```python
from build123d import *

# Parameters (mm, degrees)
SKETCH1_R           = 5.075
BOSS_EXTRUDE1_DEPTH = 20
CHAMFER1_SIZE       = 1
FILLET1_R           = 5
SKETCH2_R           = 1.5
CUT_EXTRUDE1_DEPTH  = 15
CHAMFER2_SIZE       = 1


with BuildPart() as part:
    # Sketch1 → Boss-Extrude1 (new body)
    with BuildSketch(Plane(origin=(0, 0, 0), x_dir=(0, 0, -1), z_dir=(1, 0, 0))):
        Polygon((0, 0), (60, 0), (60, 15), (45, 15), (45, 196.075), (15, 196.075), (15, 15), (0, 15), align=None)
        with Locations((30, 184.575)):
            Circle(SKETCH1_R, mode=Mode.SUBTRACT)
        with Locations((30, 167.575)):
            Circle(SKETCH1_R, mode=Mode.SUBTRACT)
    extrude(amount=BOSS_EXTRUDE1_DEPTH)

    # Chamfer1
    chamfer1_edges = [part.edges().sort_by_distance(p)[0] for p in [
        (10, 15, 0),
        (10, 196.075, -15),
        (10, 196.075, -45),
        (10, 15, -60),
    ]]
    chamfer(chamfer1_edges, length=CHAMFER1_SIZE)

    # Fillet1
    fillet1_edges = [part.edges().sort_by_distance(p)[0] for p in [
        (10, 15, -15),
        (10, 15, -45),
    ]]
    fillet(fillet1_edges, radius=FILLET1_R)

    # Sketch2 → Cut-Extrude1 (cut)
    with BuildSketch(Plane(origin=(0, 15, 0), x_dir=(1, 0, 0), z_dir=(0, 1, 0))):
        with Locations(Location((5.5, 54.5, 0), (0, 0, 270))):
            Circle(SKETCH2_R)
        with Locations(Location((14.5, 54.5, 0), (0, 0, 270))):
            Circle(SKETCH2_R)
        with Locations(Location((5.5, 5.5, 0), (0, 0, 270))):
            Circle(SKETCH2_R)
        with Locations(Location((14.5, 5.5, 0), (0, 0, 270))):
            Circle(SKETCH2_R)
    extrude(amount=-CUT_EXTRUDE1_DEPTH, mode=Mode.SUBTRACT)

    # Chamfer2
    chamfer2_edges = [part.edges().sort_by_distance(p)[0] for p in [
        (14.5, 15, -56),
        (5.5, 15, -7),
        (14.5, 15, -7),
        (5.5, 15, -56),
    ]]
    chamfer(chamfer2_edges, length=CHAMFER2_SIZE)


solid = part.part
```
Verification items for the finished model (mm, model axes). A direction names the side the tool comes from. Round coordinates to 2 decimals unless told otherwise and drop trailing zeros. Write each loop counter-clockwise with the first axis right and the second up, starting at its lowest first coordinate (ties: lowest second). Pieces come first, ordered by that corner, then holes. Notation, with made-up numbers: (89.5, 27.5) -> (140.5, 27.5) arc R5 cw to (140.5, 31.5) -> close; hole circle Ø2 at (53, 22.5). An arc over 180 degrees is marked (long way). Write each question's results on one line, items separated by ' | '. Start each with the question number.
1. Depth check by flat-ended pin: P1, Ø10, axis at x = 9, y = 142.5, coming from the -Z side; P2, Ø7, axis at x = 14, z = -53, coming from the +Y side; P3, Ø10, axis at x = 15, y = 79.5, coming from the +Z side; P4, Ø2.5, axis at x = 5.5, z = -5.5, coming from the -Y side (1 decimal). Enter the tip coordinate at first touch or a pass-through.
2. Cross-section at C-C (z = -47). Enter the section's corners in (x, y), then the cut area to 3 significant figures.
3. Set-up check for faces 1 (the flat face through (10, 106, -45)), 2 (the cylindrical face through (9.86, 179.62, -28.9)), 3 (the flat face through (10, 109, -15)): record each of +Z, -Z, +X, -X, +Y, -Y from which the full face is reachable in a straight line by a thin tool's end or side.
4. Cross-section at A-A (z = -30). Enter the section's corners in (x, y) (3 decimals), then the cut area to 3 significant figures.
5. Cross-section at B-B (y = 143). Enter the section's corners in (x, z), then the cut area to 3 significant figures.
6. Material ranges on probe 1 along Y at (x, z) = (9.75, -30) (3 decimals); probe 2 along Y at (x, z) = (1, -26.5) (3 decimals); probe 3 along X at (y, z) = (3.5, -54.5), recorded low to high. Write a range as from..to.
Solutions:
1) P1: stops at z = -45 | P2: stops at y = 15.03 | P3: stops at z = -15 | P4: passes through
2) outline: (0, 0) -> (20, 0) -> (20, 16) -> (0, 16) -> close | area: 320 mm2
3) face 1: -Z, +X, -X, +Y | face 2: +X, -X | face 3: +Z, +X, -X, +Y
4) outline: (0, 0) -> (20, 0) -> (20, 162.5) -> (0, 162.5) -> close; (0, 172.65) -> (20, 172.65) -> (20, 179.5) -> (0, 179.5) -> close; (0, 189.65) -> (20, 189.65) -> (20, 196.075) -> (0, 196.075) -> close | area: 3,520 mm2
5) outline: (0, -45) -> (20, -45) -> (20, -15) -> (0, -15) -> close | area: 600 mm2
6) probe 1: y = 0..162.5, 172.65..179.5, 189.65..196.075 | probe 2: y = 0..163.9, 171.25..180.9, 188.25..196.075 | probe 3: x = 0..4, 7..13, 16..20
